Study the drawing (mm; zero at the part's minimum x, y, z) and answer. A direction names the side the tool comes from. Round coordinates to 2 decimals unless told otherwise and drop trailing zeros. Write each loop counter-clockwise with the first axis right and the second up, starting at its lowest first coordinate (ties: lowest second). Pieces come first, ordered by that corner, then holes. Notation, with made-up numbers: (58.5, 63) - (108.5, 63) arc R12 ccw to (108.5, 74) - close; hole circle Ø7 at (-17.75, 43.5). An arc over 180 degrees is marked (long way). Use one line per item in the form item = value. Start each with the question number.
1) Each of these flat-tipped pins is pushed along its axis until it touches: pin 1 (5 mm diameter, centred on y = 4.5, z = 4, fed in from -X); pin 2 (2 mm diameter, centred on y = 5, z = 11.5, fed in from -X); pin 3 (5 mm diameter, centred on x = 4.5, z = 2.5, fed in from +Y). Where does it stop, or does it pass through?
2) For a pull along X with two mould halves and no side action, classify the marked faces 1, 2 and 3 as released by +X, released by -X, zero draft, split by the parting line, or undercut.
3) The part is cut by section A-A, the plane z = 3.5. Give the vertices of the cut face in (x, y), plus the area to 3 significant figures.
4) Consider line 1 along Z through (x, y) = (4.25, 4.5); line 2 along X through (y, z) = (2.5, 6.75); line 3 along Y through (x, z) = (2.75, 3). Determine where each line is inside the solid, lowest interval first. Write a range as from..to.
5) For the marked faces 4 and 5, determine the directions among +Z, -Z, +X, -X, +Y, -Y from which every point of the face is accessible in a straight line to the end or side of a thin tool.
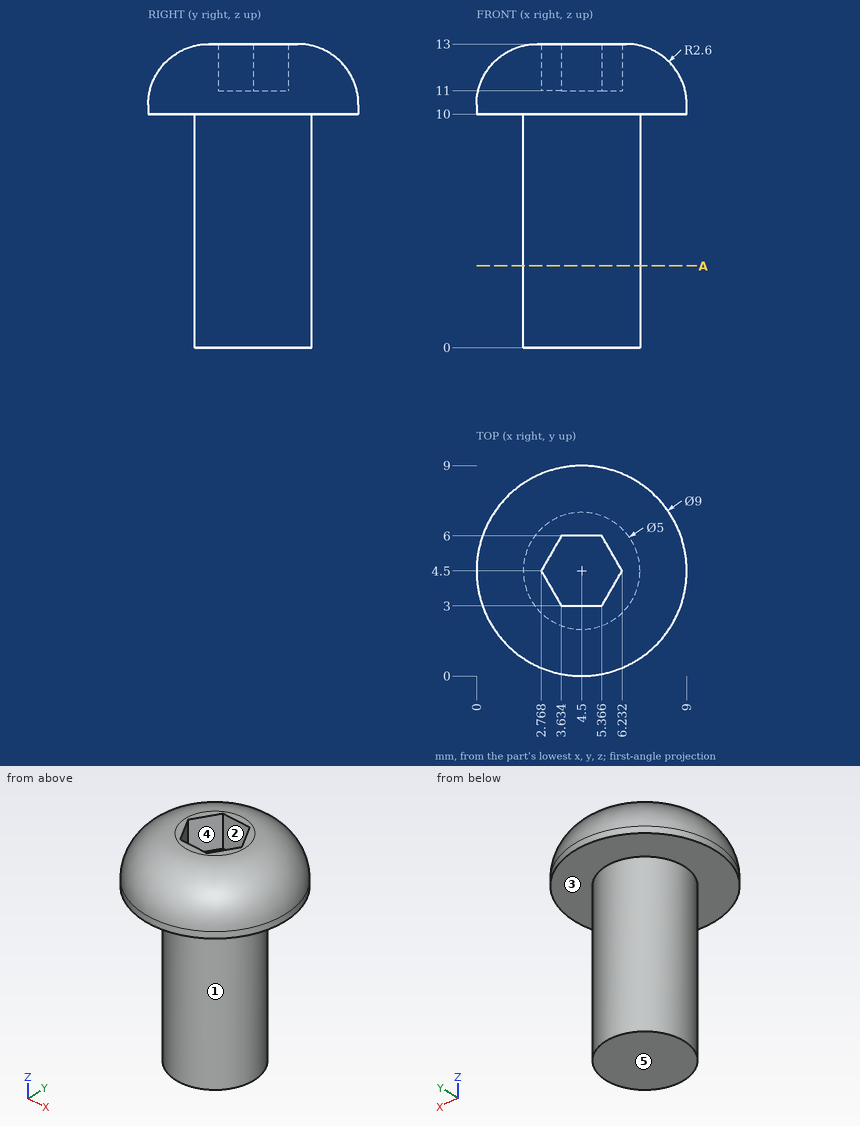
Geometry results:
q1.pin_1 = 2
q1.pin_2 = 0.01
q1.pin_3 = 7
q2.face_1 = split by the parting line
q2.face_2 = undercut
q2.face_3 = zero draft
q3.outline = circle Ø5 at (4.5, 4.5)
q3.area = 19.6 mm2
q4.line_1 = 0..11
q4.line_2 = 3..6
q4.line_3 = 2.71..6.29
q5.face_4 = +Z
q5.face_5 = -Z, +X, -X, +Y, -Y
